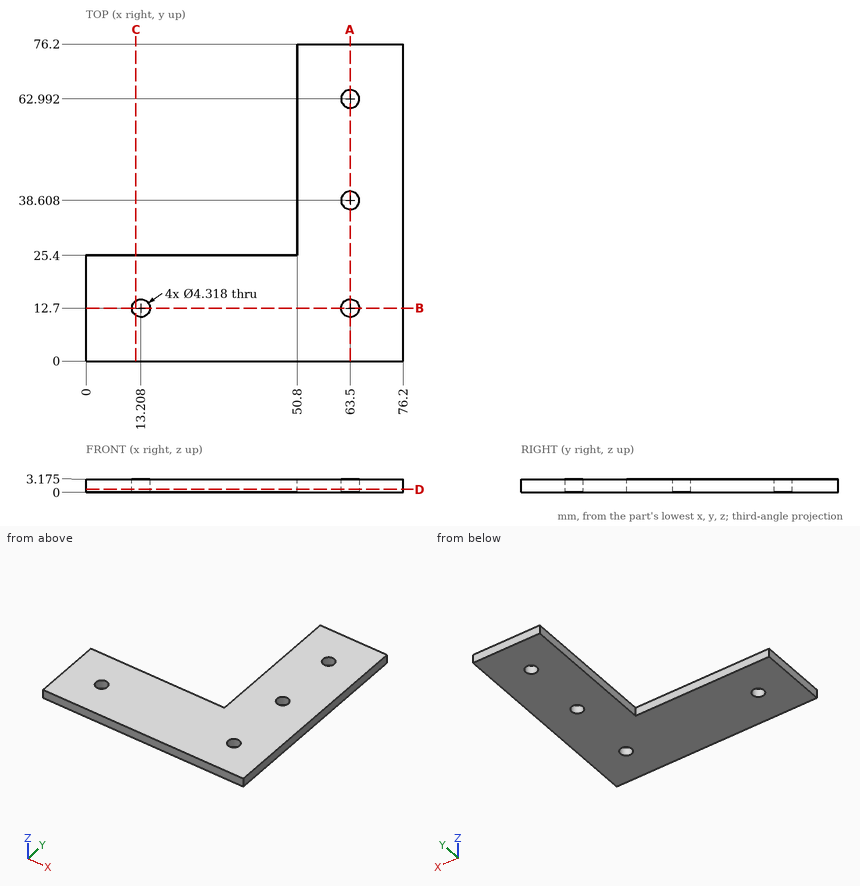
Check sheet for the drawn part. Datum: minimum x, y, z corner. Units: mm. Round coordinates to 2 decimals unless told otherwise and drop trailing zeros. Order: outer loops, then holes, each group sorted by start corner. A loop starts at its lowest first (then second) coordinate and runs counter-clockwise, first axis right, second up.
(1) Go/stop test with flat-tipped pins: P1, Ø7, axis at x = 63.5, y = 12.7, coming from the -Z side; P2, Ø1.6, axis at x = 20, z = 1.5, coming from the +Y side. Record where each tip stops, or that it passes through.
(2) Cross-section at A-A, the plane x = 63.5. Enter the section's corners in (y, z) (3 decimals), and give its area (3 significant figures).
(3) Scan lines: probe 1 along Y at (x, z) = (63.5, 2.15); probe 2 along X at (y, z) = (26, 1.7); probe 3 along Y at (x, z) = (23.5, 1). Record each from-to range of solid material in increasing order.
(4) Cross-section at B-B, the plane y = 12.7. Enter the section's corners in (x, z) (3 decimals).
(5) Cross-section at C-C, the plane x = 12. Enter the section's corners in (y, z) (3 decimals), and give its area (3 significant figures).
(6) Cross-section at D-D, the plane z = 0.7. Enter the section's corners in (x, y).
Check sheet entries:
1. P1: stops at z = 0
1. P2: stops at y = 25.4
2. outline: (0, 0) - (10.541, 0) - (10.541, 3.175) - (0, 3.175) - close; (14.859, 0) - (36.449, 0) - (36.449, 3.175) - (14.859, 3.175) - close; (40.767, 0) - (60.833, 0) - (60.833, 3.175) - (40.767, 3.175) - close; (65.151, 0) - (76.2, 0) - (76.2, 3.175) - (65.151, 3.175) - close
2. area: 201 mm2
3. probe 1: y = 0 to 10.54, 14.86 to 36.45, 40.77 to 60.83, 65.15 to 76.2
3. probe 2: x = 50.8 to 76.2
3. probe 3: y = 0 to 25.4
4. outline: (0, 0) - (11.049, 0) - (11.049, 3.175) - (0, 3.175) - close; (15.367, 0) - (61.341, 0) - (61.341, 3.175) - (15.367, 3.175) - close; (65.659, 0) - (76.2, 0) - (76.2, 3.175) - (65.659, 3.175) - close
5. outline: (0, 0) - (10.911, 0) - (10.911, 3.175) - (0, 3.175) - close; (14.489, 0) - (25.4, 0) - (25.4, 3.175) - (14.489, 3.175) - close
5. area: 69.3 mm2
6. outline: (0, 0) - (76.2, 0) - (76.2, 76.2) - (50.8, 76.2) - (50.8, 25.4) - (0, 25.4) - close; hole circle Ø4.32 at (13.21, 12.7); hole circle Ø4.32 at (63.5, 12.7); hole circle Ø4.32 at (63.5, 38.61); hole circle Ø4.32 at (63.5, 62.99)
